Can you work these out from the model? Positions are in its coordinate system, mm. Face numbers are marked on the shaded views. Round coordinates to 2 decimals unless told otherwise and drop trailing zeros. Loops run counter-clockwise (first coordinate to the right, second up) from the corner with the lowest first, then second, coordinate; pieces in that order, holes last. Notation, with made-up numbers: (-34, 78.5) -> (11, 78.5) arc R15 cw to (11, 93.5) -> close; hole circle Ø9 at (-23, 70.25). An arc over 180 degrees is marked (long way). Write each question's results on one line, items separated by ' | '.
Autodesk Inventor part; units mm, degrees
ref_plane "YZ Plane" through (0, 0, 0) normal (1, 0, 0) x (0, 1, 0)
ref_plane "XZ Plane" through (0, 0, 0) normal (0, 1, 0) x (-1, 0, 0)
ref_plane "XY Plane" through (0, 0, 0) normal (0, 0, 1) x (1, 0, 0)
sketch "Sketch1" plane through (0, 0, 0) normal (0, 0, 1) x (1, 0, 0)
  line L0 (-35, 35) -> (35, 35)
  line L1 (35, 35) -> (35, -35)
  line L2 (35, -35) -> (-35, -35)
  line L3 (-35, -35) -> (-35, 35)
  point P0 (0, 0)
  dimension "d0" = 70
  dimension "d1" = 70
  dimension "d2" = 35
  dimension "d3" = 35
extrude "Extrusion1" add sketch "Sketch1" along normal blind 8
sketch "Sketch2" plane through (0, 0, 8) normal (0, 0, 1) x (1, 0, 0)
  line L0 (-35, 35) -> (-35, -35)
  line L1 (-35, 27) -> (-30, 27)
  line L2 (-30, 27) -> (-30, 17)
  line L3 (-30, 17) -> (-35, 17)
  line L4 (-35, 17) -> (-35, 27)
  line L5 (35, 35) -> (-35, 35)
  line L6 (0, -49) -> (0, 49)
  line L7 (35, 27) -> (30, 27)
  line L8 (30, 27) -> (30, 17)
  line L9 (30, 17) -> (35, 17)
  line L10 (35, 17) -> (35, 27)
  line L11 (-49, 0) -> (49, 0)
  line L12 (-35, -27) -> (-30, -27)
  line L13 (-30, -27) -> (-30, -17)
  line L14 (-30, -17) -> (-35, -17)
  line L15 (-35, -17) -> (-35, -27)
  line L16 (30, -17) -> (35, -17)
  line L17 (30, -27) -> (30, -17)
  line L18 (35, -27) -> (30, -27)
  line L19 (35, -17) -> (35, -27)
  point P0 (0, 0)
  dimension "d7" = 10
  dimension "d8" = 8
  dimension "d9" = 5
extrude "Extrusion2" add sketch "Sketch2" along normal blind 10 contours L14 L13 L12 L0 | L1 L2 L3 L0 | L10 L9 L8 L7 | L16 L19 L18 L17
sketch "Sketch3" plane through (-35, -35, 0) normal (-1, 0, 0) x (0, 0, 1)
  line L0 (8, 62) -> (8, 52)
  line L1 (18, 62) -> (18, 52)
  line L2 (8, 62) -> (18, 62)
  line L3 (8, 52) -> (18, 52)
  line L4 (8, 18) -> (8, 8)
  line L5 (8, 18) -> (18, 18)
  line L6 (8, 8) -> (18, 8)
  line L7 (18, 18) -> (18, 8)
  circle A0 centre (13, 57) radius 2.5
  circle A1 centre (13, 13) radius 2.5
  point P0 (0, 35)
  dimension "d12" = 5
  dimension "d13" = 5
  dimension "d14" = 5
  dimension "d15" = 5
  dimension "d17" = 5
extrude "Extrusion3" cut sketch "Sketch3" against normal through all contours A0 | A1
equation "\"d1\" = d0"
equation "\"d8\" = width"
equation "\"width\" = 8"
properties part number "steven_example"
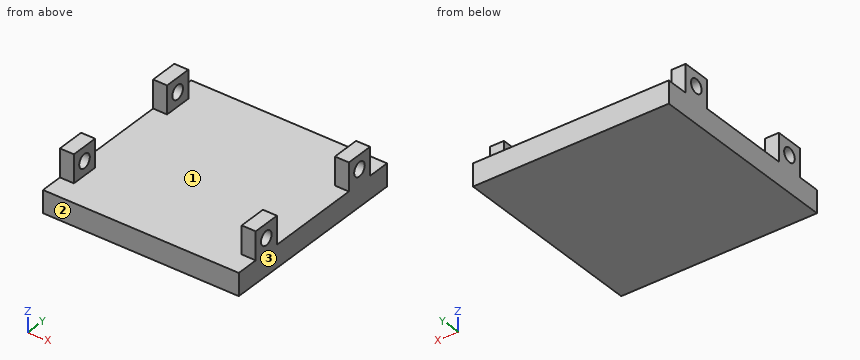
1. Please list where these lines run through material, in increasing order: line 1 (Y direction, x = -33.75, z = 13); line 2 (Z direction, x = 7, y = 26.5). Write a range as from..to.
Final values:
line 1: -27..-24.5, -19.5..-17, 17..19.5, 24.5..27 | line 2: 0..8
2. We'd pull the mould along X, two halves only. Please class the marked faces 1, 2 and 3: pulls with the +X half, pulls with the -X half, needs draft (parallel to the pull), parting line crosses it, or undercut.
Final values:
face 1: undercut | face 2: needs draft | face 3: pulls with the +X half
3. Will these pins go through, and if not, where does the flat tip stop? pin 1 (4 mm diameter, centred on x = 31.5, z = 15, fed in from +Y); pin 2 (5 mm diameter, centred on y = -27.5, z = 13.5, fed in from +X); pin 3 (5.5 mm diameter, centred on x = 33.5, z = 15, fed in from -Y); pin 4 (3 mm diameter, centred on x = -23, y = 19.5, fed in from +Z).
Final values:
pin 1: y = 27 | pin 2: x = 35 | pin 3: y = -27 | pin 4: z = 8
4. If we section it at D-D (x = 10): List the corners of the cut face in (y, z) for me, then the cut area to 3 significant figures.
Final values:
outline: (-35, 0) -> (35, 0) -> (35, 8) -> (-35, 8) -> close | area: 560 mm2
5. If we section it at C-C (z = 13): State how many separate pieces and enclosed holes the cut face has, then the cut area to 3 significant figures.
Final values:
separate pieces: 8 | enclosed holes: 0 | area: 100 mm2
6. If we section it at B-B (y = -22): List the corners of the cut face in (x, z) for me, then the cut area to 3 significant figures.
Final values:
outline: (-35, 0) -> (35, 0) -> (35, 10.5) -> (30, 10.5) -> (30, 8) -> (-30, 8) -> (-30, 10.5) -> (-35, 10.5) -> close; (-35, 15.5) -> (-30, 15.5) -> (-30, 18) -> (-35, 18) -> close; (30, 15.5) -> (35, 15.5) -> (35, 18) -> (30, 18) -> close | area: 610 mm2
7. If we section it at A-A (z = 9.25): List the corners of the cut face in (x, y) for me, then the cut area to 3 significant figures.
Final values:
outline: (-35, -27) -> (-30, -27) -> (-30, -17) -> (-35, -17) -> close; (-35, 17) -> (-30, 17) -> (-30, 27) -> (-35, 27) -> close; (30, -27) -> (35, -27) -> (35, -17) -> (30, -17) -> close; (30, 17) -> (35, 17) -> (35, 27) -> (30, 27) -> close | area: 200 mm2
